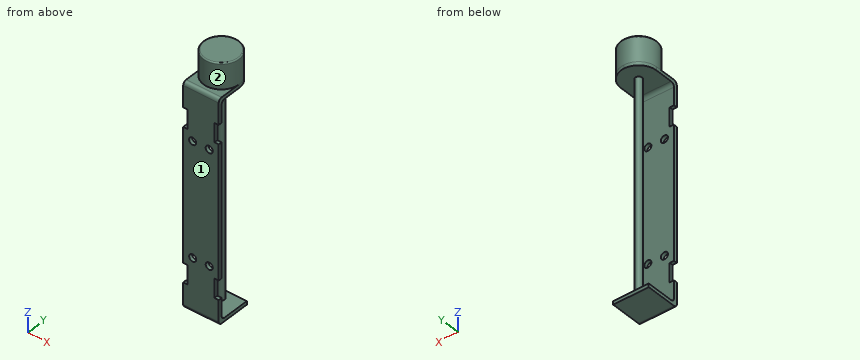
from build123d import *

# Parameters (mm, degrees)
BOSS_EXTRU_1_DEPTH      = 15
CONG_1_R                = 1.5
ESQUISSE2_R             = 7.5
BOSS_EXTRU_2_DEPTH      = 10.8
CONG_2_R                = 7.5
ESQUISSE3_R             = 1.5
ESQUISSE3_W             = 1.8
ESQUISSE3_H             = 8
ENL_V_MAT_EXTRU_1_DEPTH = 62.905492487
ESQUISSE4_R             = 1.45
BOSS_EXTRU_3_DEPTH      = 90
CONG_3_R                = 0.5


with BuildPart() as part:
    # Esquisse1 → Boss.-Extru.1 (new body)
    with BuildSketch(Plane(origin=(0, 0, 0), x_dir=(0, 0, -1), z_dir=(1, 0, 0))):
        Polygon((-46.5, 0), (46.5, 0), (46.5, 14.5), (45, 14.5), (45, 1.5), (-45, 1.5), (-45, 18), (-46.5, 18), align=None)
    extrude(amount=BOSS_EXTRU_1_DEPTH)

    # Congé1
    cong_1_edges = [part.edges().sort_by_distance(p)[0] for p in [
        (7.5, 1.5, 45),
        (7.5, 1.5, -45),
        (7.5, 0, -46.5),
        (7.5, 0, 46.5),
    ]]
    fillet(cong_1_edges, radius=CONG_1_R)

    # Esquisse2 → Boss.-Extru.2 (add)
    with BuildSketch(Plane.XY.offset(46.5)):
        with Locations((7.5, 10.5)):
            Circle(ESQUISSE2_R)
    extrude(amount=BOSS_EXTRU_2_DEPTH)

    # Congé2
    cong_2_edges = [part.edges().sort_by_distance(p)[0] for p in [
        (0, 18, 45.75),
        (15, 18, 45.75),
    ]]
    fillet(cong_2_edges, radius=CONG_2_R - 0.0001)  # a hair under: the kernel refuses the full size

    # Esquisse3 → Enlèv. mat.-Extru.1 (cut, through all)
    with BuildSketch(Plane.XZ):
        with Locations(Location((4, 24, 0), (0, 0, 270))):
            Circle(ESQUISSE3_R)
        with Locations(Location((11, 24, 0), (0, 0, 270))):
            Circle(ESQUISSE3_R)
        with Locations(Location((4, -24, 0), (0, 0, 270))):
            Circle(ESQUISSE3_R)
        with Locations(Location((11, -24, 0), (0, 0, 270))):
            Circle(ESQUISSE3_R)
        with Locations((0.9, 32)):
            Rectangle(ESQUISSE3_W, ESQUISSE3_H)
        with Locations((14.1, 32)):
            Rectangle(ESQUISSE3_W, ESQUISSE3_H)
        with Locations((14.1, -32)):
            Rectangle(ESQUISSE3_W, ESQUISSE3_H)
        with Locations((0.9, -32)):
            Rectangle(ESQUISSE3_W, ESQUISSE3_H)
    extrude(amount=-ENL_V_MAT_EXTRU_1_DEPTH, mode=Mode.SUBTRACT)

    # Esquisse4 → Boss.-Extru.3 (add)
    with BuildSketch(Plane(origin=(0, 0, 45), x_dir=(-1, 0, 0), z_dir=(0, 0, -1))):
        with Locations(Location((-7.5, 10.5, 0), (0, 0, 180))):
            Circle(ESQUISSE4_R)
    extrude(amount=BOSS_EXTRU_3_DEPTH)

    # Congé3
    cong_3_edges = [part.edges().sort_by_distance(p)[0] for p in [
        (0, 10.5, 57.3),
    ]]
    fillet(cong_3_edges, radius=CONG_3_R)


solid = part.part
Design review of the part built by this model. Coordinates are the model's own, in mm. Face numbers are marked on the shaded views. A direction names the side the tool comes from. Coordinates: 2 decimals unless noted, no trailing zeros. Loops run counter-clockwise (first coordinate to the right, second up) from the corner with the lowest first, then second, coordinate; pieces in that order, holes last. Notation, with made-up numbers: (69.5, 44) - (90.5, 44) arc R15 cw to (90.5, 68) - close; hole circle Ø1 at (57, 73.5). An arc over 180 degrees is marked (long way). Use CSV: the item, a comma, the result in double quotes. Start each with the question number.
1. Clearance check with flat-ended pins moving along their axes: pin 1 (4 mm diameter, centred on x = 11, z = -24, fed in from +Y); pin 2 (1.5 mm diameter, centred on x = 11, z = -34.5, fed in from -Y); pin 3 (1.2 mm diameter, centred on y = 0.5, z = 31.5, fed in from +X); pin 4 (0.8 mm diameter, centred on x = 1, y = 1, fed in from -Z). State where each tip first meets the part, or that it passes through.
2. To check wall thickness, follow probe 1 along X at (y, z) = (0.45, 24); probe 2 along Z at (x, y) = (10, 11.75); probe 3 along Z at (x, y) = (2.25, 2.75). State the ranges of each line that lie inside material, in increasing order.
3. Add section A-A on z = -24. Give the boundary of the cut face in (x, y), plus the area to 3 significant figures.
4. Add section C-C on x = 4. Count the separate pieces of the cut face and the enclosed holes in it, plus the area to 3 significant figures.
5. Add section B-B on z = 38. Give the boundary of the cut face in (x, y), plus the area to 3 significant figures.
6. For the marked faces 1 and 2, list the 3-axis set-ups (+Z, -Z, +X, -X, +Y, -Y) from which the entire face can be reached by the end or side of a thin tool; tool diameter is ignored.
Resolved:
1,pin 1,"y = 1.5"
1,pin 2,"y = 0"
1,pin 3,"x = 13.2"
1,pin 4,"z = -46.5"
2,probe 1,"0 to 2.5, 5.5 to 9.5, 12.5 to 15"
2,probe 2,"-46.5 to -45, 45 to 57.3"
2,probe 3,"-46.5 to -44.98, 44.98 to 46.5"
3,outline,"(0, 0) - (2.5, 0) - (2.5, 1.5) - (0, 1.5) - close; (5.5, 0) - (9.5, 0) - (9.5, 1.5) - (5.5, 1.5) - close; circle Ø2.9 at (7.5, 10.5); (12.5, 0) - (15, 0) - (15, 1.5) - (12.5, 1.5) - close"
3,area,"20.1 mm2"
4,separate pieces,"3"
4,enclosed holes,"0"
4,area,"317 mm2"
5,outline,"(0, 0) - (15, 0) - (15, 1.5) - (0, 1.5) - close; circle Ø2.9 at (7.5, 10.5)"
5,area,"29.1 mm2"
6,face 1,"+Z, -Z, +X, -X, -Y"
6,face 2,"+Z"
